The listing builds one solid part. Answer for the finished solid, in the listing's coordinates (mm). Face numbers are marked on the shaded views. Coordinates: 2 decimals unless noted, no trailing zeros. Write each loop counter-clockwise with the first axis right and the second up, starting at its lowest first coordinate (ties: lowest second). Pieces come first, ordered by that corner, then holes.
```python
from build123d import *

# Parameters (mm, degrees)
BOSS_EXTRUDE1_DEPTH = 76.2
BOSS_EXTRUDE1_TAPER = 4.5
SHELL1_T            = -3.302
SKETCH3_R           = 2.667
CUT_EXTRUDE1_DEPTH  = 94.3255592
FILLET1_R           = 2.54


with BuildPart() as part:
    # Sketch1 → Boss-Extrude1 (new body)
    with BuildSketch(Plane.XY):
        Polygon((19.05, 38.1), (0, 0), (38.1, 0), align=None)
    extrude(amount=BOSS_EXTRUDE1_DEPTH, taper=BOSS_EXTRUDE1_TAPER)

    # Shell1
    shell1_openings = [part.faces().sort_by_distance(p)[0] for p in [
        (19.05, 2.656988988, 33.76024606),
    ]]
    offset(amount=SHELL1_T, openings=shell1_openings, kind=Kind.INTERSECTION)

    # Sketch3 → Cut-Extrude1 (cut, through all)
    with BuildSketch(Plane(origin=(0, 0, 0), x_dir=(0, 0, -1), z_dir=(1, 0, 0))):
        with Locations(Location((-66.04, 14.114950363, 0), (0, 0, 279.98084931))):
            Circle(SKETCH3_R)
    extrude(amount=CUT_EXTRUDE1_DEPTH, mode=Mode.SUBTRACT)

    # Fillet1
    # the kernel refuses this fillet: 2.54 mm, written as the material it takes off along each edge
    with BuildSketch(Plane(origin=(39.379699759, -0.790897947, -10.049311237), x_dir=(-0.9920380235210648, -0.00988103768125179, -0.12555048778384248), z_dir=(-0.12593871481168567, 0.07783440625310155, 0.9889799013705022)), Plane(origin=(-1.279699759, -0.790897947, -10.049311237), x_dir=(0.43481502259412097, 0.8917247171317577, -0.1255504877838424), z_dir=(0.1259387148116856, 0.07783440625310152, 0.9889799013705022))) as fillet1_piece_1:
        with BuildLine():
            CenterArc((FILLET1_R * 1.60020309461, -FILLET1_R), FILLET1_R, 90, 115.995770326)
            Line((FILLET1_R * 0.701376689441, -FILLET1_R * 1.43830479506), (0, 0))
            Line((0, 0), (FILLET1_R * 1.60020309461, 0))
        make_face()
    extrude(amount=97.371667857, mode=Mode.SUBTRACT)
    with BuildSketch(Plane(origin=(19.05, 40.267836366, -12.318486277), x_dir=(-0.45268605430468506, -0.8781752040708111, -0.1545433505306691), z_dir=(0, -0.1733190032733758, 0.9848657386183782))) as fillet1_piece_2:
        with BuildLine():
            CenterArc((FILLET1_R * 1.96973147724, FILLET1_R), FILLET1_R, 143.832298895, 126.167701105)
            Line((FILLET1_R * 1.16243835589, FILLET1_R * 1.59015067248), (0, 0))
            Line((0, 0), (FILLET1_R * 1.96973147724, 0))
        make_face()
    extrude(amount=102.386529419, mode=Mode.SUBTRACT)


solid = part.part
```
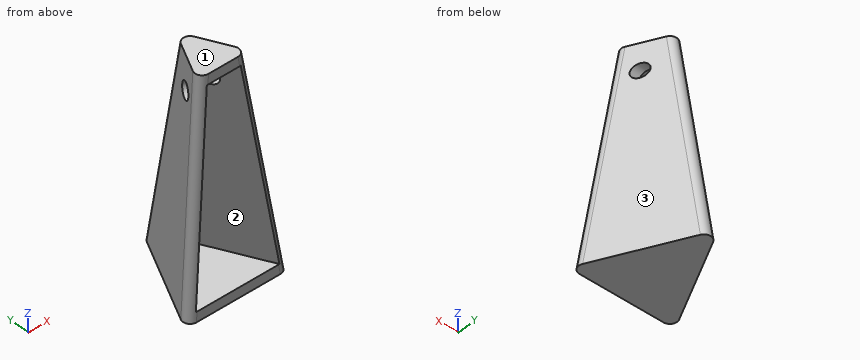
(1) Section B-B, the plane z = 66.5 is taken. State how many separate pieces and enclosed holes the cut face has, plus the area to 3 significant figures.
(2) Each of these flat-tipped pins is pushed along its axis until it touches: pin 1 (1 mm diameter, centred on y = 26.5, z = 10, fed in from -X); pin 2 (5 mm diameter, centred on x = 18.5, z = 10.5, fed in from -Y); pin 3 (8.5 mm diameter, centred on y = 14.11, z = 66.04, fed in from -X). Where does it stop, or does it pass through?
(3) Section A-A, the plane y = 14 is taken. Write down the section's boundary in (x, z).
(4) Find the intervals of material crossed by probe 1 along Z at (x, y) = (19.5, 8); probe 2 along X at (y, z) = (3, 24.5); probe 3 along X at (y, z) = (9.5, 62.5), in increasing order.
(5) For a pull along X with two mould halves and no side action, classify the marked faces 1, 2 and 3 as pulls with the +X half, pulls with the -X half, needs draft (parallel to the pull), parting line crosses it, or undercut.
Solution:
1. separate pieces: 3
1. enclosed holes: 0
1. area: 77.0 mm2
2. pin 1: stops at x = 13.88
2. pin 2: stops at y = 22.73
2. pin 3: stops at x = 10.71
3. outline: (7, 0) - (31.1, 0) - (25.52, 63.38) - (21.82, 63.38) - (27.11, 3.3) - (10.99, 3.3) - (16.28, 63.38) - (12.58, 63.38) - close; (13.05, 68.7) - (16.75, 68.7) - (17.12, 72.9) - (20.98, 72.9) - (21.35, 68.7) - (25.05, 68.7) - (24.4, 76.2) - (13.7, 76.2) - close
4. probe 1: z = 0 to 3.3, 72.9 to 76.2
4. probe 2: x = 5.14 to 7.36, 30.74 to 32.96
4. probe 3: x = 10.25 to 13.95, 24.15 to 27.85
5. face 1: needs draft
5. face 2: undercut
5. face 3: pulls with the +X half
